```python
from build123d import *

# Parameters (mm, degrees)
F3_SIZE  = 1.27
F5_D     = 5.1054
F5_DEPTH = 29.21
F5_TIP   = 1.5338169022


# Not quite as in the source:
# - a fillet or chamfer that OpenCascade refuses, or shapes differently, is made with other operations: its cross-section is extruded or revolved along the edge and cut away or added


with BuildPart() as f1:
    # F0 (on Front) → F1 (revolve)
    with BuildSketch(Plane.XZ):
        Polygon((9.525, 12.7), (0, 12.7), (0, -31.75), (6.35, -31.75), (6.35, 0), (9.525, 0), align=None)
    revolve(axis=Axis((0, 0, -3.4719856316), (0, 0, -1)))

    # F2: fillet of radius 5.08 on 2 edges, made by hand

    # F2_s1 → F2_t2 (revolve, cut)
    with BuildSketch(Plane.XZ):
        with BuildLine():
            ThreePointArc((4.445, 12.7), (8.0371024484, 11.2121024484), (9.525, 7.62))
            Line((9.525, 7.62), (9.525, 12.7))
            Line((9.525, 12.7), (4.445, 12.7))
        make_face()
    revolve(axis=Axis((0, 0, 12.7), (0, 0, -1)), mode=Mode.SUBTRACT)

    # F2_s3 → F2_t4 (revolve, cut)
    with BuildSketch(Plane.XZ):
        with BuildLine():
            ThreePointArc((6.35, 0), (8.6571134838, 1.8694797079), (9.525, 4.7092860393))
            Line((9.525, 4.7092860393), (9.525, 0))
            Line((9.525, 0), (6.35, 0))
        make_face()
    revolve(axis=Axis((0, 0, 0), (0, 0, -1)), mode=Mode.SUBTRACT)

    # F3
    f3_edges = [f1.edges().sort_by_distance(p)[0] for p in [
        (-6.35, 0, -31.75),
    ]]
    chamfer(f3_edges, length=F3_SIZE)

    # F5
    with Locations(Plane(origin=(0, 0, -31.75), x_dir=(1, 0, 0), z_dir=(0, 0, -1))):
        with Locations((0, 0)):
            Hole(F5_D / 2, depth=F5_DEPTH)
            with Locations((0, 0, -(F5_DEPTH + F5_TIP / 2))):  # 118° drill point
                Cone(0, F5_D / 2, F5_TIP, mode=Mode.SUBTRACT)


solid = f1.part
```
The model under review builds one solid part; all positions refer to its coordinate system, in mm. Round coordinates to 2 decimals unless told otherwise and drop trailing zeros. Order: outer loops, then holes, each group sorted by start corner. A loop starts at its lowest first (then second) coordinate and runs counter-clockwise, first axis right, second up.
Item 1: To check wall thickness, follow probe 1 along Y at (x, z) = (0, -15.25); probe 2 along Z at (x, y) = (-4.25, -1.5); probe 3 along Z at (x, y) = (3.25, -8). State the ranges of each line that lie inside material, in increasing order.
Working result:
probe 1: y = -6.35 to -2.55, 2.55 to 6.35
probe 2: z = -31.75 to 12.7
probe 3: z = 1.84 to 10.49
Item 2: For pin 1 (6 mm diameter, centred on y = 4.5, z = 7.5, fed in from +X); pin 2 (5 mm diameter, centred on y = 1, z = -14, fed in from -X); pin 3 (5 mm diameter, centred on x = 6, y = 7, fed in from -Z), all flat-tipped, find the tip position at first contact; note any pin that passes through.
Working result:
pin 1: stops at x = 9.41
pin 2: stops at x = -6.35
pin 3: stops at z = 0.17
Item 3: Draft analysis for pull direction X (two halves, no side actions). For faces 1 (the conical face through (0.42, -0.13, -1.27)), 2 (the flat face through (0, 0, 12.7)), 3 (the cylindrical face through (-2.435, -0.767, -16.941)), 4 (the cylindrical face through (-1.38, 6.2, -15.03)), state which applies: released by +X, released by -X, zero draft, split by the parting line, or undercut.
Working result:
face 1: undercut
face 2: zero draft
face 3: undercut
face 4: split by the parting line
Item 4: Add section B-B, the plane z = -0.5. State the section outline as (x, y) points.
Working result:
outline: circle Ø12.7 at (0, 0)
Item 5: Add section A-A, the plane z = -22. State the section outline as (x, y) points.
Working result:
outline: circle Ø12.7 at (0, 0); hole circle Ø5.11 at (0, 0)
